Here's how the part is built. I have some questions about the finished solid (model axes, mm). Face numbers are marked on the shaded views. A direction names the side the tool comes from. Coordinates: 2 decimals unless noted, no trailing zeros. Loops run counter-clockwise (first coordinate to the right, second up) from the corner with the lowest first, then second, coordinate; pieces in that order, holes last. Notation, with made-up numbers: (73, 34.5) -> (123, 34.5) arc R35 cw to (123, 69.5) -> close; hole circle Ø10 at (28, -8). An arc over 180 degrees is marked (long way). Answer as a JSON object with one key per item and string values. Group by question number.
Q1. On a 3-axis mill with a long thin cutter (end or side, diameter ignored), from which of +Z, -Z, +X, -X, +Y, -Y can I reach the whole of each face in a straight line? I mean the marked faces 4, 5, 6 and 7. Say none if no direction works.
Q2. I'm going to push flat-ended pins straight in: pin 1 (10 mm diameter, centred on y = 31, z = 9.5, fed in from +X); pin 2 (3 mm diameter, centred on x = -4, y = 20, fed in from +Z); pin 3 (3.5 mm diameter, centred on x = -11, y = 29.5, fed in from -Z). Where does each tip first touch, or does it pass through?
Q3. Thinking about a two-plate mould opening in Z: for the marked faces 1, 2 and 3, which applies, released by +Z, released by -Z, zero draft, split by the parting line, or undercut?
Q4. I want a section at C-C on x = 0. Write out the boundary of the cut face in (y, z) (3 decimals), then the cut area to 3 significant figures.
Q5. I need wall thicknesses on line 1 (Z direction, x = 0, y = 13) (3 decimals); line 2 (Z direction, x = 11, y = 46); line 3 (Z direction, x = -5, y = 48). Which ranges of each line are inside material? Lowest first, please.
Q6. I want a section at A-A on x = 10. Write out the boundary of the cut face in (y, z).
Q7. I want a section at B-B on z = 0. Write out the boundary of the cut face in (x, y) (3 decimals).
Q8. I want a section at D-D on y = 30. Write out the boundary of the cut face in (x, z) (3 decimals).
```python
from build123d import *

# Parameters (mm, degrees)
SKETCH1_R      = 0.825
EXTRUDE1_DEPTH = 54


with BuildPart() as part:
    # Sketch1 → Extrude1 (new body)
    with BuildSketch(Plane(origin=(0, 0, 0), x_dir=(1, 0, 0), z_dir=(0, 1, 0))):
        with BuildLine():
            Line((-2.945413127, 12.957690258), (-3.288294978, 9.038532772))
            ThreePointArc((-3.288294978, 9.038532772), (-4.250108449, 7.08816799), (-6.276879072, 6.3))
            Line((-6.276879072, 6.3), (-13.625, 6.3))
            ThreePointArc((-13.625, 6.3), (-19.925, 0), (-13.625, -6.3))
            Line((-13.625, -6.3), (-6.666750968, -6.3))
            ThreePointArc((-6.666750968, -6.3), (-4.639980345, -7.08816799), (-3.678166874, -9.038532772))
            Line((-3.678166874, -9.038532772), (-3.332323508, -12.99154053))
            ThreePointArc((-3.332323508, -12.99154053), (0, -16.045052443), (3.332323508, -12.99154053))
            Line((3.332323508, -12.99154053), (3.678166874, -9.038532772))
            ThreePointArc((3.678166874, -9.038532772), (4.639980345, -7.08816799), (6.666750968, -6.3))
            Line((6.666750968, -6.3), (13.625, -6.3))
            ThreePointArc((13.625, -6.3), (19.925, 0), (13.625, 6.3))
            Line((13.625, 6.3), (6.276879072, 6.3))
            ThreePointArc((6.276879072, 6.3), (4.250108449, 7.08816799), (3.288294978, 9.038532772))
            Line((3.288294978, 9.038532772), (2.945413127, 12.957690258))
            ThreePointArc((2.945413127, 12.957690258), (0, 15.656664127), (-2.945413127, 12.957690258))
        make_face()
        with Locations((0, 12.7)):
            Circle(SKETCH1_R, mode=Mode.SUBTRACT)
        with Locations((0, -12.7)):
            Circle(SKETCH1_R, mode=Mode.SUBTRACT)
        with BuildLine():
            Line((-13.625, 4.75), (13.625, 4.75))
            ThreePointArc((13.625, 4.75), (18.375, 0), (13.625, -4.75))
            Line((13.625, -4.75), (-13.625, -4.75))
            ThreePointArc((-13.625, -4.75), (-18.375, 0), (-13.625, 4.75))
        make_face(mode=Mode.SUBTRACT)
    extrude(amount=EXTRUDE1_DEPTH)


solid = part.part
```
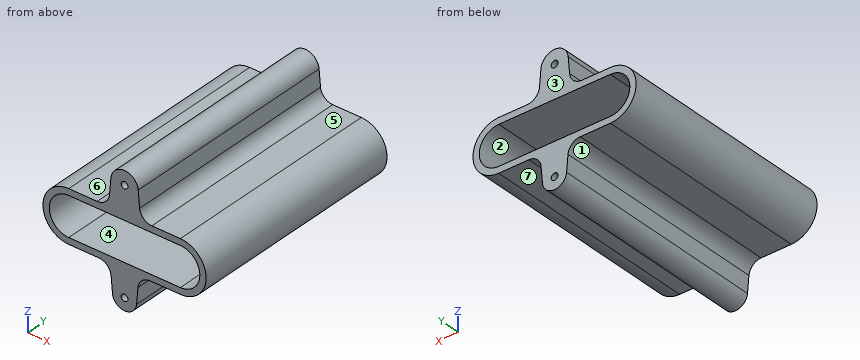
Result set:
{
 "1": {"face 4": "+Y, -Y", "face 5": "+Z, +X, +Y, -Y", "face 6": "+Z, -X, +Y, -Y", "face 7": "-Z, +X, +Y, -Y"},
 "2": {"pin 1": "stops at x = 18.03", "pin 2": "stops at z = 14.92", "pin 3": "stops at z = -6.3"},
 "3": {"face 1": "released by -Z", "face 2": "undercut", "face 3": "zero draft"},
 "4": {"outline": "(0, -15.657) -> (54, -15.657) -> (54, -13.525) -> (0, -13.525) -> close; (0, -11.875) -> (54, -11.875) -> (54, -4.75) -> (0, -4.75) -> close; (0, 4.75) -> (54, 4.75) -> (54, 11.875) -> (0, 11.875) -> close; (0, 13.525) -> (54, 13.525) -> (54, 16.045) -> (0, 16.045) -> close", "area": "1,020 mm²"},
 "5": {"line 1": "z = -15.657 to -13.525, -11.875 to -4.75, 4.75 to 11.875, 13.525 to 16.045", "line 2": "z = -6.3 to -4.75, 4.75 to 6.3", "line 3": "z = -6.59 to -4.75, 4.75 to 6.81"},
 "6": {"outline": "(0, -6.3) -> (54, -6.3) -> (54, -4.75) -> (0, -4.75) -> close; (0, 4.75) -> (54, 4.75) -> (54, 6.3) -> (0, 6.3) -> close"},
 "7": {"outline": "(-19.925, 0) -> (-18.375, 0) -> (-18.375, 54) -> (-19.925, 54) -> close; (18.375, 0) -> (19.925, 0) -> (19.925, 54) -> (18.375, 54) -> close"},
 "8": {"outline": "(-13.625, -6.3) -> (-6.277, -6.3) arc R3 cw to (-3.288, -9.039) -> (-2.945, -12.958) arc R2.957 ccw to (2.945, -12.958) -> (3.288, -9.039) arc R3 cw to (6.277, -6.3) -> (13.625, -6.3) arc R6.3 ccw to (13.625, 6.3) -> (6.667, 6.3) arc R3 cw to (3.678, 9.039) -> (3.332, 12.992) arc R3.345 ccw to (-3.332, 12.992) -> (-3.678, 9.039) arc R3 cw to (-6.667, 6.3) -> (-13.625, 6.3) arc R6.3 ccw to start; hole (-13.625, -4.75) -> (13.625, -4.75) arc R4.75 ccw to (13.625, 4.75) -> (-13.625, 4.75) arc R4.75 ccw to start; hole circle Ø1.65 at (0, -12.7); hole circle Ø1.65 at (0, 12.7)"}
}
